Verification items for this drawing (mm, ordinates from the low corner). Round coordinates to 2 decimals unless told otherwise and drop trailing zeros. Loops run counter-clockwise (first coordinate to the right, second up) from the corner with the lowest first, then second, coordinate; pieces in that order, holes last. Notation, with made-up numbers: M 53.5,31.25 L 71.5,31.25 A23 ccw 71.5,54.25 Z; hole C -20.75,79 d10. An arc over 180 degrees is marked long. Answer as CSV lines item,"result".
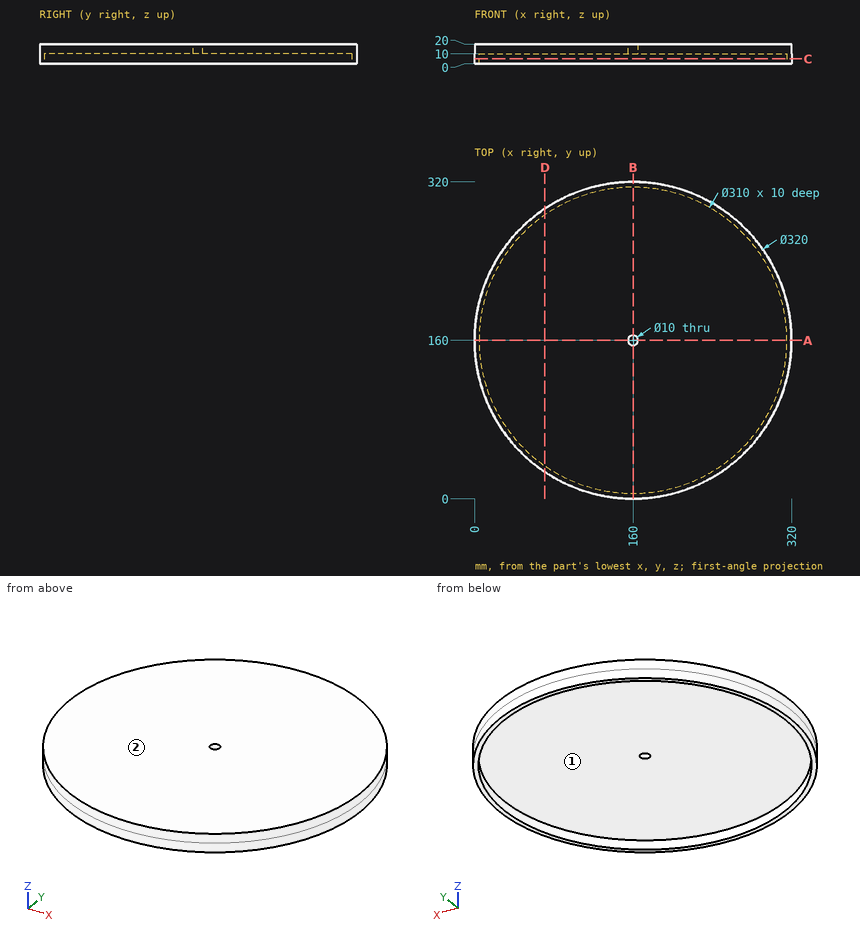
1) Section check D-D (x = 71). Record the cut outline in (y, z), plus the area to 3 significant figures.
Here are the results:
outline,"M 27.04,0 L 33.1,0 L 33.1,10 L 286.9,10 L 286.9,0 L 292.96,0 L 292.96,20 L 27.04,20 Z"
area,"2,780 mm^2"
2) Material ranges on probe 1 along Y at (x, z) = (160, 3.25); probe 2 along Y at (x, z) = (163.5, 3); probe 3 along Z at (x, y) = (176, 135), recorded low to high.
Here are the results:
probe 1,"y = 0 to 5, 315 to 320"
probe 2,"y = 0.04 to 5.04, 314.96 to 319.96"
probe 3,"z = 10 to 20"
3) Draft check along X on the marked faces 1 and 2. Enter one of: +X half, -X half, draft (parallel to the pull), parting line (faces both ways), or undercut.
Here are the results:
face 1,"undercut"
face 2,"draft"
4) Section check A-A (y = 160). Record the cut outline in (x, z).
Here are the results:
outline,"M 0,0 L 5,0 L 5,10 L 155,10 L 155,20 L 0,20 Z; M 165,10 L 315,10 L 315,0 L 320,0 L 320,20 L 165,20 Z"
5) Section check C-C (z = 5). Record the cut outline in (x, y).
Here are the results:
outline,"C 160,160 d320; hole C 160,160 d310"
6) Go/stop test with flat-tipped pins: pin 1 (1 mm diameter, centred on y = 45, z = 12.5, fed in from -X); pin 2 (6 mm diameter, centred on x = 136, y = 188, fed in from -Z); pin 3 (1.5 mm diameter, centred on x = 100.5, z = 5, fed in from -Y). Record where each tip stops, or that it passes through.
Here are the results:
pin 1,"stops at x = 48.24"
pin 2,"stops at z = 10"
pin 3,"stops at y = 11.18"
